from build123d import *

# Parameters (mm, degrees)
F0_W     = 246
F0_H     = 429
F1_DEPTH = 12
F2_SIZE  = 11.99999
F4_D     = 3.5


# Not quite as in the source:
# - a fillet or chamfer is up to 0.001 mm smaller than in the source, because OpenCascade refuses the exact size
# - a feature names something its author has since deleted; it is built from what else it names


with BuildPart() as f1:
    # F0 (on Front) → F1 (new body)
    with BuildSketch(Plane.XZ):
        Rectangle(F0_W, F0_H)
    extrude(amount=F1_DEPTH)

    # F2 (size 12 in the source; OpenCascade refuses exactly that, so slightly less here)
    f2_edges = [f1.edges().sort_by_distance(p)[0] for p in [
        (123, 0, 0),
        (0, 0, 214.5),
        (-123, 0, 0),
    ]]
    chamfer(f2_edges, length=F2_SIZE)

    # F4 (through all)
    with Locations(Plane.XZ.offset(12)):
        with Locations((-90.5, 195), (90.5, 195), (-90.5, -157), (90.5, -157)):
            Hole(F4_D / 2)


solid = f1.part
Check sheet for the modelled part. Datum: model origin and axes. Units: mm. Give positions to 0.01 mm unless a question says otherwise; leave off trailing zeros. Order: outer loops, then holes, each group sorted by start corner. A loop starts at its lowest first (then second) coordinate and runs counter-clockwise, first axis right, second up. Notation, with made-up numbers: (51, 23) - (94, 23) arc R11 ccw to (94, 32) - close; hole circle Ø11 at (32, 15.25). An arc over 180 degrees is marked (long way). Answer as CSV lines item,"result".
1. Scan lines: probe 1 along X at (y, z) = (-8.25, 195); probe 2 along Z at (x, y) = (-90.5, -6.5); probe 3 along Z at (x, y) = (-90.5, -4). Record each from-to range of solid material in increasing order. Write a range as from..to.
Result sheet:
probe 1,"-119.25..-92.25, -88.75..88.75, 92.25..119.25"
probe 2,"-214.5..-158.75, -155.25..193.25, 196.75..209"
probe 3,"-214.5..-158.75, -155.25..193.25, 196.75..206.5"
2. Go/stop test with flat-tipped pins: P1, Ø2, axis at x = 80.5, y = -6, coming from the +Z side; P2, Ø3, axis at y = -9.5, z = 90.5, coming from the -X side; P3, Ø4, axis at y = -2, z = -95, coming from the +X side. Record where each tip stops, or that it passes through.
Result sheet:
P1,"z = 209.5"
P2,"x = -122"
P3,"x = 115"
3. Section check A-A (y = -2.25). Record the boundary of the cut face in (x, z).
Result sheet:
outline,"(-113.25, -214.5) - (113.25, -214.5) - (113.25, 204.75) - (-113.25, 204.75) - close; hole circle Ø3.5 at (-90.5, -157); hole circle Ø3.5 at (-90.5, 195); hole circle Ø3.5 at (90.5, -157); hole circle Ø3.5 at (90.5, 195)"
